```python
from build123d import *

# Parameters (mm, degrees)
SKETCH_1_W           = 250
SKETCH_1_H           = 29
SKETCH_1_W_2         = 30
SKETCH_1_H_2         = 15
EXTRUDE_1_DEPTH      = 28
SKETCH_1_3_R         = 2
CUT_EXTRUDE_1_DEPTH  = 132.450561049
CUT_EXTRUDE_START    = 2
SKETCH_1_5_R         = 2
CUT_EXTRUDE_2_DEPTH  = 24
SKETCH_3_W           = 6
SKETCH_3_H           = 19
EXTRUDE_2_DEPTH      = 35
SKETCH_3_3_W         = 6
SKETCH_3_3_H         = 19
EXTRUDE_3_DEPTH      = 35
SKETCH_1_6_R         = 2
CUT_EXTRUDE_3_DEPTH  = 166.088612569
CUT_EXTRUDE_7_REACH  = 167.089
SKETCH_1_8_R         = 3.1
FILLET_1_R           = 9.5
FILLET_2_R           = 5
SKETCH_4_R           = 5.1
CUT_EXTRUDE_4_DEPTH  = 31.5
SKETCH_4_2_OUTSIDE_W = 87.946
SKETCH_4_2_OUTSIDE_H = 103.946
SKETCH_4_2_OUTSIDE_R = 5.1
CUT_EXTRUDE_5_DEPTH  = 21.5
SKETCH_5_OUTSIDE_W   = 83.722
SKETCH_5_OUTSIDE_H   = 99.722
SKETCH_5_OUTSIDE_W_2 = 23.8
SKETCH_5_OUTSIDE_H_2 = 24.8
CUT_EXTRUDE_6_DEPTH  = 18
SKETCH_6_R           = 0.75
CUT_EXTRUDE_8_DEPTH  = 4
SKETCH_7_R           = 0.75
CUT_EXTRUDE_9_DEPTH  = 4
SKETCH_8_R           = 0.75
CUT_EXTRUDE_10_DEPTH = 4
SKETCH_9_R           = 0.75
CUT_EXTRUDE_11_DEPTH = 4
SKETCH_11_R          = 0.75
CUT_EXTRUDE_12_DEPTH = 166.088612569
CUT_EXTRUDE_13_DEPTH = 166.088612569
CUT_EXTRUDE_START_2  = 30
SKETCH_13_W          = 20.2
SKETCH_13_H          = 21.2
CUT_EXTRUDE_14_DEPTH = 40
SKETCH_11_5_R        = 1.5
CUT_EXTRUDE_18_DEPTH = 112.204766085
SKETCH_11_6_R        = 2.25
CUT_EXTRUDE_19_DEPTH = 2
CUT_EXTRUDE_START_3  = 26
SKETCH_11_7_R        = 2.25
CUT_EXTRUDE_20_DEPTH = 2
SKETCH_15_W          = 16
SKETCH_15_H          = 2.5
SKETCH_15_H_2        = 10
CUT_EXTRUDE_21_DEPTH = 3


with BuildPart() as part:
    # 草图1 → 凸台-拉伸1 (new body)
    with BuildSketch(Plane(origin=(0, 0, 0), x_dir=(0, 0, -1), z_dir=(1, 0, 0))):
        Rectangle(SKETCH_1_W, SKETCH_1_H)
        with Locations((-60, 22)):
            Rectangle(SKETCH_1_W_2, SKETCH_1_H_2)
        with Locations((0, 22)):
            Rectangle(SKETCH_1_W_2, SKETCH_1_H_2)
        with Locations((60, 22)):
            Rectangle(SKETCH_1_W_2, SKETCH_1_H_2)
    extrude(amount=EXTRUDE_1_DEPTH)

    # 草图1<3> → 切除-拉伸1 (cut, through all)
    with BuildSketch(Plane(origin=(0, 0, 0), x_dir=(0, 0, -1), z_dir=(1, 0, 0))):
        with Locations((-67.5, -10.858617882)):
            Circle(SKETCH_1_3_R)
        with Locations((-22.5, -10.858617882)):
            Circle(SKETCH_1_3_R)
        with Locations((22.5, -10.858617882)):
            Circle(SKETCH_1_3_R)
        with Locations((-60, 25.5)):
            Circle(SKETCH_1_3_R)
        with Locations((67.5, -10.858617882)):
            Circle(SKETCH_1_3_R)
        with Locations((0, 25.5)):
            Circle(SKETCH_1_3_R)
        with Locations((60, 25.5)):
            Circle(SKETCH_1_3_R)
    extrude(amount=CUT_EXTRUDE_1_DEPTH, mode=Mode.SUBTRACT)

    # 草图1<5> → 切除-拉伸2 (cut)
    # profile 1 of 7: a face of its own
    with BuildSketch(Plane(origin=(0, 0, 0), x_dir=(0, 0, -1), z_dir=(1, 0, 0)).offset(CUT_EXTRUDE_START)):
        with BuildLine():
            Line((-72.5, 29.5), (-72.5, 25.5))
            ThreePointArc((-72.5, 25.5), (-60, 13), (-47.5, 25.5))
            Line((-47.5, 25.5), (-47.5, 29.5))
            Line((-47.5, 29.5), (-72.5, 29.5))
        make_face()
        with Locations((-60, 25.5)):
            Circle(SKETCH_1_5_R, mode=Mode.SUBTRACT)
    # profile 2 of 7: a face of its own
    with BuildSketch(Plane(origin=(0, 0, 0), x_dir=(0, 0, -1), z_dir=(1, 0, 0)).offset(CUT_EXTRUDE_START)):
        with BuildLine():
            Line((-79.457856675, -14.5), (-55.542143325, -14.5))
            ThreePointArc((-55.542143325, -14.5), (-67.5, 1.641382118), (-79.457856675, -14.5))
        make_face()
        with Locations((-67.5, -10.858617882)):
            Circle(SKETCH_1_5_R, mode=Mode.SUBTRACT)
    # profile 3 of 7: a face of its own
    with BuildSketch(Plane(origin=(0, 0, 0), x_dir=(0, 0, -1), z_dir=(1, 0, 0)).offset(CUT_EXTRUDE_START)):
        with BuildLine():
            Line((-34.457856675, -14.5), (-10.542143325, -14.5))
            ThreePointArc((-10.542143325, -14.5), (-22.5, 1.641382118), (-34.457856675, -14.5))
        make_face()
        with Locations((-22.5, -10.858617882)):
            Circle(SKETCH_1_5_R, mode=Mode.SUBTRACT)
    # profile 4 of 7: a face of its own
    with BuildSketch(Plane(origin=(0, 0, 0), x_dir=(0, 0, -1), z_dir=(1, 0, 0)).offset(CUT_EXTRUDE_START)):
        with BuildLine():
            ThreePointArc((-12.5, 25.5), (0, 13), (12.5, 25.5))
            Line((12.5, 25.5), (12.5, 29.5))
            Line((12.5, 29.5), (-12.5, 29.5))
            Line((-12.5, 29.5), (-12.5, 25.5))
        make_face()
        with Locations((0, 25.5)):
            Circle(SKETCH_1_5_R, mode=Mode.SUBTRACT)
    # profile 5 of 7: a face of its own
    with BuildSketch(Plane(origin=(0, 0, 0), x_dir=(0, 0, -1), z_dir=(1, 0, 0)).offset(CUT_EXTRUDE_START)):
        with BuildLine():
            Line((10.542143325, -14.5), (34.457856675, -14.5))
            ThreePointArc((34.457856675, -14.5), (22.5, 1.641382118), (10.542143325, -14.5))
        make_face()
        with Locations((22.5, -10.858617882)):
            Circle(SKETCH_1_5_R, mode=Mode.SUBTRACT)
    # profile 6 of 7: a face of its own
    with BuildSketch(Plane(origin=(0, 0, 0), x_dir=(0, 0, -1), z_dir=(1, 0, 0)).offset(CUT_EXTRUDE_START)):
        with BuildLine():
            Line((55.542143325, -14.5), (79.457856675, -14.5))
            ThreePointArc((79.457856675, -14.5), (67.5, 1.641382118), (55.542143325, -14.5))
        make_face()
        with Locations((67.5, -10.858617882)):
            Circle(SKETCH_1_5_R, mode=Mode.SUBTRACT)
    # profile 7 of 7: a face of its own
    with BuildSketch(Plane(origin=(0, 0, 0), x_dir=(0, 0, -1), z_dir=(1, 0, 0)).offset(CUT_EXTRUDE_START)):
        with BuildLine():
            ThreePointArc((47.5, 25.5), (60, 13), (72.5, 25.5))
            Line((72.5, 25.5), (72.5, 29.5))
            Line((72.5, 29.5), (47.5, 29.5))
            Line((47.5, 29.5), (47.5, 25.5))
        make_face()
        with Locations((60, 25.5)):
            Circle(SKETCH_1_5_R, mode=Mode.SUBTRACT)
    extrude(amount=CUT_EXTRUDE_2_DEPTH, mode=Mode.SUBTRACT)

    # 草图3 → 凸台-拉伸2 (add)
    with BuildSketch(Plane.XY.offset(125)):
        with Locations((25, 0)):
            Rectangle(SKETCH_3_W, SKETCH_3_H)
    extrude(amount=EXTRUDE_2_DEPTH)

    # 草图3<3> → 凸台-拉伸3 (add)
    with BuildSketch(Plane.XY.offset(125)):
        with Locations((25, 0)):
            Rectangle(SKETCH_3_3_W, SKETCH_3_3_H)
        with Locations((3, 0)):
            Rectangle(SKETCH_3_3_W, SKETCH_3_3_H)
    extrude(amount=EXTRUDE_3_DEPTH)

    # 草图1<6> → 切除-拉伸3 (cut, through all)
    with BuildSketch(Plane(origin=(0, 0, 0), x_dir=(0, 0, -1), z_dir=(1, 0, 0))):
        with Locations(Location((-150, 0, 0), (0, 0, 90))):
            Circle(SKETCH_1_6_R)
    extrude(amount=CUT_EXTRUDE_3_DEPTH, mode=Mode.SUBTRACT)

    # 草图1<8> → 切除-拉伸7 (cut, up to next)
    with BuildSketch(Plane(origin=(0, 0, 0), x_dir=(0, 0, -1), z_dir=(1, 0, 0)), mode=Mode.PRIVATE) as cut_extrude_7_sk1:
        with Locations(Location((-150, 0, 0), (0, 0, 180))):
            Circle(SKETCH_1_8_R)
    cut_extrude_7_tool1 = extrude(cut_extrude_7_sk1.sketch, amount=CUT_EXTRUDE_7_REACH, mode=Mode.PRIVATE) & part.part
    add(cut_extrude_7_tool1.solids().sort_by_distance((0, 0, 150))[0], mode=Mode.SUBTRACT)

    # 圆角1
    fillet_1_edges = [part.edges().sort_by_distance(p)[0] for p in [
        (25, 9.5, 160),
        (25, -9.5, 160),
        (3, -9.5, 160),
        (3, 9.5, 160),
    ]]
    fillet(fillet_1_edges, radius=FILLET_1_R - 0.0001)  # a hair under: the kernel refuses the full size

    # 圆角2
    fillet_2_edges = [part.edges().sort_by_distance(p)[0] for p in [
        (14, -14.5, 125),
        (14, 14.5, 125),
    ]]
    fillet(fillet_2_edges, radius=FILLET_2_R)

    # 草图4 → 切除-拉伸4 (cut)
    with BuildSketch(Plane(origin=(0, 0, -125), x_dir=(-1, 0, 0), z_dir=(0, 0, -1))):
        with Locations((-14, 0)):
            Circle(SKETCH_4_R)
    extrude(amount=-CUT_EXTRUDE_4_DEPTH, mode=Mode.SUBTRACT)

    # 草图4<2> outside → 切除-拉伸5 (cut)
    with BuildSketch(Plane(origin=(0, 0, -125), x_dir=(-1, 0, 0), z_dir=(0, 0, -1))):
        with Locations((-14, 7.5)):
            Rectangle(SKETCH_4_2_OUTSIDE_W, SKETCH_4_2_OUTSIDE_H)
        with Locations((-14, 0)):
            Circle(SKETCH_4_2_OUTSIDE_R, mode=Mode.SUBTRACT)
    extrude(amount=-CUT_EXTRUDE_5_DEPTH, mode=Mode.SUBTRACT)

    # 草图5 outside → 切除-拉伸6 (cut)
    with BuildSketch(Plane(origin=(0, 0, -103.5), x_dir=(-1, 0, 0), z_dir=(0, 0, -1))):
        with Locations((-14, 7.5)):
            Rectangle(SKETCH_5_OUTSIDE_W, SKETCH_5_OUTSIDE_H)
        with Locations((-14, 0)):
            Rectangle(SKETCH_5_OUTSIDE_W_2, SKETCH_5_OUTSIDE_H_2, mode=Mode.SUBTRACT)
    extrude(amount=-CUT_EXTRUDE_6_DEPTH, mode=Mode.SUBTRACT)

    # 草图6 → 切除-拉伸8 (cut)
    with BuildSketch(Plane(origin=(0, 14.5, 0), x_dir=(1, 0, 0), z_dir=(0, 1, 0))):
        with Locations(Location((7, 23.5, 0), (0, 0, 270))):
            Circle(SKETCH_6_R)
        with Locations(Location((21, 35.5, 0), (0, 0, 270))):
            Circle(SKETCH_6_R)
        with Locations(Location((7, -23.5, 0), (0, 0, 270))):
            Circle(SKETCH_6_R)
        with Locations(Location((21, -35.5, 0), (0, 0, 270))):
            Circle(SKETCH_6_R)
    extrude(amount=-CUT_EXTRUDE_8_DEPTH, mode=Mode.SUBTRACT)

    # 草图7 → 切除-拉伸9 (cut)
    with BuildSketch(Plane(origin=(0, 14.5, 0), x_dir=(1, 0, 0), z_dir=(0, 1, 0))):
        with Locations(Location((7, -89.5, 0), (0, 0, 270))):
            Circle(SKETCH_7_R)
        with Locations(Location((21.2, -110.5, 0), (0, 0, 270))):
            Circle(SKETCH_7_R)
    extrude(amount=-CUT_EXTRUDE_9_DEPTH, mode=Mode.SUBTRACT)

    # 草图8 → 切除-拉伸10 (cut)
    with BuildSketch(Plane.ZY):
        with Locations((47, 4)):
            Circle(SKETCH_8_R)
        with Locations((2.499047641, -1.5)):
            Circle(SKETCH_8_R)
    extrude(amount=-CUT_EXTRUDE_10_DEPTH, mode=Mode.SUBTRACT)

    # 草图9 → 切除-拉伸11 (cut)
    with BuildSketch(Plane(origin=(28, 0, 0), x_dir=(0, 0, -1), z_dir=(1, 0, 0))):
        with Locations((-107.5, -0.5)):
            Circle(SKETCH_9_R)
        with Locations((-92.5, -0.5)):
            Circle(SKETCH_9_R)
    extrude(amount=-CUT_EXTRUDE_11_DEPTH, mode=Mode.SUBTRACT)

    # 草图11 → 切除-拉伸12 (cut, through all)
    with BuildSketch(Plane(origin=(0, 0, 0), x_dir=(0, 0, -1), z_dir=(1, 0, 0))):
        with Locations((-14.530122053, 6.5)):
            Circle(SKETCH_11_R)
        with Locations((-1.081846191, -6.5)):
            Circle(SKETCH_11_R)
        with Locations((5.469877947, 6.5)):
            Circle(SKETCH_11_R)
    extrude(amount=CUT_EXTRUDE_12_DEPTH, mode=Mode.SUBTRACT)

    # 草图10 → 切除-拉伸13 (cut, through all)
    with BuildSketch(Plane.ZY):
        Polygon((30, 14.5), (0, -14.5), (0, -65.636075395), (207.45026546, -65.636075395), (207.45026546, 45.542128626), (30, 45.542128626), align=None)
    extrude(amount=-CUT_EXTRUDE_13_DEPTH, mode=Mode.SUBTRACT)

    # 草图13 → 切除-拉伸14 (cut)
    with BuildSketch(Plane.XY.offset(CUT_EXTRUDE_START_2)):
        with Locations((14, 0)):
            Rectangle(SKETCH_13_W, SKETCH_13_H)
    extrude(amount=-CUT_EXTRUDE_14_DEPTH, mode=Mode.SUBTRACT)

    # 草图11<5> → 切除-拉伸18 (cut, through all)
    with BuildSketch(Plane(origin=(0, 0, 0), x_dir=(0, 0, -1), z_dir=(1, 0, 0))):
        with Locations(Location((-14.530122053, 6.5, 0), (0, 0, 90))):
            Circle(SKETCH_11_5_R)
        with Locations(Location((-1.081846191, -6.5, 0), (0, 0, 90))):
            Circle(SKETCH_11_5_R)
        with Locations(Location((5.469877947, 6.5, 0), (0, 0, 90))):
            Circle(SKETCH_11_5_R)
    extrude(amount=CUT_EXTRUDE_18_DEPTH, mode=Mode.SUBTRACT)

    # 草图11<6> → 切除-拉伸19 (cut)
    with BuildSketch(Plane(origin=(0, 0, 0), x_dir=(0, 0, -1), z_dir=(1, 0, 0))):
        with Locations((-14.530122053, 6.5)):
            Circle(SKETCH_11_6_R)
        with Locations((-1.081846191, -6.5)):
            Circle(SKETCH_11_6_R)
        with Locations((5.469877947, 6.5)):
            Circle(SKETCH_11_6_R)
    extrude(amount=CUT_EXTRUDE_19_DEPTH, mode=Mode.SUBTRACT)

    # 草图11<7> → 切除-拉伸20 (cut)
    with BuildSketch(Plane(origin=(0, 0, 0), x_dir=(0, 0, -1), z_dir=(1, 0, 0)).offset(CUT_EXTRUDE_START_3)):
        with Locations((-14.530122053, 6.5)):
            Circle(SKETCH_11_7_R)
        with Locations((-1.081846191, -6.5)):
            Circle(SKETCH_11_7_R)
        with Locations((5.469877947, 6.5)):
            Circle(SKETCH_11_7_R)
    extrude(amount=CUT_EXTRUDE_20_DEPTH, mode=Mode.SUBTRACT)

    # 草图15 → 切除-拉伸21 (cut)
    with BuildSketch(Plane(origin=(0, 29.5, 0), x_dir=(1, 0, 0), z_dir=(0, 1, 0))):
        with Locations((14, 73.75)):
            Rectangle(SKETCH_15_W, SKETCH_15_H)
        with Locations((14, 71.25)):
            Rectangle(SKETCH_15_W, SKETCH_15_H)
        with Locations((14, 65)):
            Rectangle(SKETCH_15_W, SKETCH_15_H_2)
    extrude(amount=-CUT_EXTRUDE_21_DEPTH, mode=Mode.SUBTRACT)


solid = part.part
```
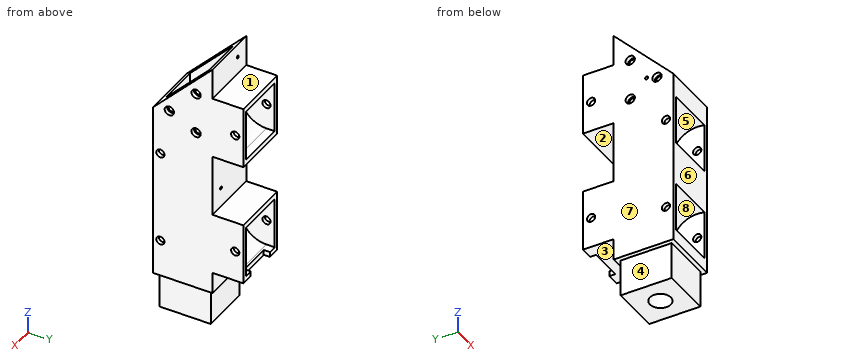
Geometry check sheet. Reference: the model listing, model coordinates, mm. Face numbers are marked on the shaded views. A direction names the side the tool comes from. Coordinates: 2 decimals unless noted, no trailing zeros. Order: outer loops, then holes, each group sorted by start corner. A loop starts at its lowest first (then second) coordinate and runs counter-clockwise, first axis right, second up. Notation, with made-up numbers: M 44,77.5 L 50,77.5 A17 cw 50,90.5 Z; hole C -34,82 d7. An arc over 180 degrees is marked long. Answer as a JSON object with one key per item and string values.
Q1. Cross-section at B-B on z = -78. Record the cut outline in (x, y).
Results are:
{"outline": "M 0,-14.5 L 2,-14.5 L 2,-4.08 L 26,-4.08 L 26,-14.5 L 28,-14.5 L 28,14.5 L 0,14.5 Z"}
Q2. Tool access check on the marked faces 1, 2, 3 and 4. Record the directions out of +Z, -Z, +X, -X, +Y, -Y that give a thin tool (end or side, any length) a straight path to the whole face; none if there is none.
Results are:
{"face 1": "+Z, +X, -X, +Y", "face 2": "+X, -X, +Y", "face 3": "-Z, +X, -X, +Y", "face 4": "-Z, -X, +Y, -Y"}
Q3. Cross-section at C-C on y = 6.5. Give the number of separate pieces and of enclosed holes in the cut face, and give its area (3 significant figures).
Results are:
{"separate pieces": "5", "enclosed holes": "0", "area": "2,730 mm²"}
Q4. Release check for a two-part mould opening along X. For the marked faces 5, 6, 7 and 8 record: released by +X, released by -X, zero draft, split by the parting line, or undercut.
Results are:
{"face 5": "undercut", "face 6": "zero draft", "face 7": "released by -X", "face 8": "undercut"}
Q5. Cross-section at A-A on z = -60. Record the cut outline in (x, y), and give its area (3 significant figures).
Results are:
{"outline": "M 0,-14.5 L 2,-14.5 L 2,-0.86 L 26,-0.86 L 26,-14.5 L 28,-14.5 L 28,23.5 L 26,23.5 L 26,13 L 2,13 L 2,23.5 L 0,23.5 Z; M 0,27.5 L 2,27.5 L 2,29.5 L 0,29.5 Z; M 26,27.5 L 28,27.5 L 28,29.5 L 26,29.5 Z", "area": "493 mm²"}
Q6. Scan lines: line 1 (Z direction, x = 24.95, y = 6.5); line 2 (Y direction, x = 27, z = -60); line 3 (Z direction, x = 12.25, y = -2). Record each from-to range of solid material in increasing order.
Results are:
{"line 1": "z = -103.5 to -6.97, -3.97 to 13.03, 16.03 to 21.72", "line 2": "y = -14.5 to 23.5, 27.5 to 29.5", "line 3": "z = -93.5 to -76.32, -58.68 to -31.32, -13.68 to -10"}
Q7. Depth check by flat-ended pin: pin 1 Ø1.2 at (x, y) = (18, 28) entering from -Z; pin 2 Ø1 at (x, z) = (13, -69.5) entering from -Y; pin 3 Ø4.5 at (x, y) = (10, 28) entering from +Z. Enter the tip coordinate at first touch or a pass-through.
Results are:
{"pin 1": "stops at z = -47.5", "pin 2": "stops at y = 1.39", "pin 3": "stops at z = 15"}
